The model under review builds one solid part; all positions refer to its coordinate system, in mm. Face numbers are marked on the shaded views. Round coordinates to 2 decimals unless told otherwise and drop trailing zeros.
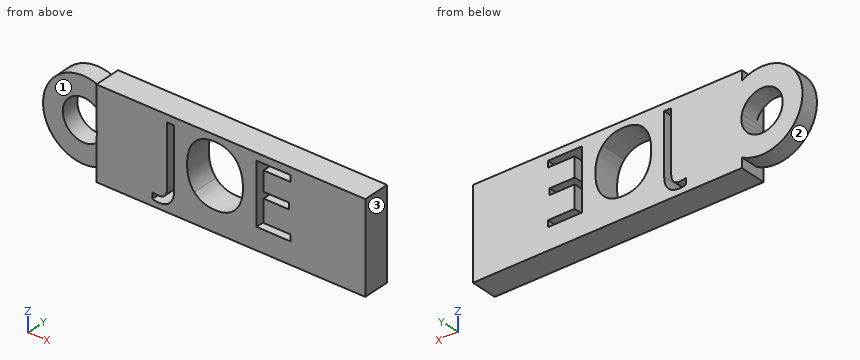
```python
from build123d import *

# Parameters (mm, degrees)
F1_DEPTH = 15
F2_DEPTH = 10


with BuildPart() as f1:
    # F0 (on Front) → F1 (new body)
    with BuildSketch(Plane.XZ):
        with BuildLine():
            Line((-150, 0), (0, 0))
            Line((0, 0), (0, 50))
            Line((0, 50), (-150, 50))
            Line((-150, 50), (-150, 44.6036947758))
            Line((-150, 44.6036947758), (-150, 27.5289733242))
            ThreePointArc((-150, 27.5289733242), (-149.78939418, 26.2722736231), (-149.7189046187, 25))
            ThreePointArc((-149.7189046187, 25), (-149.78939418, 23.7277263769), (-150, 22.4710266758))
            Line((-150, 22.4710266758), (-150, 5.3963052242))
            Line((-150, 5.3963052242), (-150, 0))
        make_face()
        with BuildLine():
            add(Edge.make_bspline(
                [(-108.8792543819, 5.5825479955), (-111.1049800612, 3.1602165479), (-115.2819252527, 3.1602165479)],
                knots=[0, 0, 0, 1, 1, 1], degree=2))
            add(Edge.make_bspline(
                [(-115.2819252527, 3.1602165479), (-117.4557173328, 3.1602165479), (-118.7095427989, 3.7834197381)],
                knots=[0, 0, 0, 1, 1, 1], degree=2))
            Line((-118.7095427989, 3.7834197381), (-118.7095427989, 7.1442655139))
            add(Edge.make_bspline(
                [(-118.7095427989, 7.1442655139), (-117.0625057962, 6.6842822068), (-115.2819252527, 6.6842822068)],
                knots=[0, 0, 0, 1, 1, 1], degree=2))
            add(Edge.make_bspline(
                [(-115.2819252527, 6.6842822068), (-112.9820087174, 6.6842822068), (-111.7875359362, 8.0753607564)],
                knots=[0, 0, 0, 1, 1, 1], degree=2))
            add(Edge.make_bspline(
                [(-111.7875359362, 8.0753607564), (-110.593063155, 9.4664393059), (-110.593063155, 12.0853765219)],
                knots=[0, 0, 0, 1, 1, 1], degree=2))
            Line((-110.593063155, 12.0853765219), (-110.593063155, 45.9831786178))
            Line((-110.593063155, 45.9831786178), (-106.6535287026, 45.9831786178))
            Line((-106.6535287026, 45.9831786178), (-106.6535287026, 12.4118162882))
            add(Edge.make_bspline(
                [(-106.6535287026, 12.4118162882), (-106.6535287026, 8.0048794432), (-108.8792543819, 5.5825479955)],
                knots=[0, 0, 0, 1, 1, 1], degree=2))
        make_face(mode=Mode.SUBTRACT)
        with BuildLine():
            add(Edge.make_bspline(
                [(-72.3402578132, 41.8804242823), (-68.2375034777, 37.2434957837), (-68.2375034777, 29.0825016263)],
                knots=[0, 0, 0, 1, 1, 1], degree=2))
            add(Edge.make_bspline(
                [(-68.2375034777, 29.0825016263), (-68.2375034777, 20.9437647256), (-72.3550959844, 16.2808694274)],
                knots=[0, 0, 0, 1, 1, 1], degree=2))
            add(Edge.make_bspline(
                [(-72.3550959844, 16.2808694274), (-76.4726884911, 11.6179741293), (-83.7953259761, 11.6179741293)],
                knots=[0, 0, 0, 1, 1, 1], degree=2))
            add(Edge.make_bspline(
                [(-83.7953259761, 11.6179741293), (-91.2811833442, 11.6179741293), (-95.3505517945, 16.1992594859)],
                knots=[0, 0, 0, 1, 1, 1], degree=2))
            add(Edge.make_bspline(
                [(-95.3505517945, 16.1992594859), (-99.4199202448, 20.7805448424), (-99.4199202448, 29.1270161398)],
                knots=[0, 0, 0, 1, 1, 1], degree=2))
            add(Edge.make_bspline(
                [(-99.4199202448, 29.1270161398), (-99.4199202448, 37.4067156669), (-95.3394231661, 41.9620342239)],
                knots=[0, 0, 0, 1, 1, 1], degree=2))
            add(Edge.make_bspline(
                [(-95.3394231661, 41.9620342239), (-91.2589260874, 46.5173527809), (-83.7508114625, 46.5173527809)],
                knots=[0, 0, 0, 1, 1, 1], degree=2))
            add(Edge.make_bspline(
                [(-83.7508114625, 46.5173527809), (-76.4430121488, 46.5173527809), (-72.3402578132, 41.8804242823)],
                knots=[0, 0, 0, 1, 1, 1], degree=2))
        make_face(mode=Mode.SUBTRACT)
        Polygon((-41.7884633219, 15.6094421808), (-41.7884633219, 12.0853765219), (-60.6848743392, 12.0853765219), (-60.6848743392, 45.9831786178), (-41.7884633219, 45.9831786178), (-41.7884633219, 42.4813702157), (-56.7453398869, 42.4813702157), (-56.7453398869, 31.5604762159), (-42.6935917648, 31.5604762159), (-42.6935917648, 28.0809250706), (-56.7453398869, 28.0809250706), (-56.7453398869, 15.6094421808), align=None, mode=Mode.SUBTRACT)
    extrude(amount=F1_DEPTH)

    # F0 (on Front) → F2 (join)
    with BuildSketch(Plane.XZ):
        with BuildLine():
            ThreePointArc((-150, 44.6036947758), (-183.8311862448, 25), (-150, 5.3963052242))
            Line((-150, 5.3963052242), (-150, 22.4710266758))
            ThreePointArc((-150, 22.4710266758), (-172.7527967389, 25), (-150, 27.5289733242))
            Line((-150, 27.5289733242), (-150, 44.6036947758))
        make_face()
    extrude(amount=F2_DEPTH)


solid = f1.part
```
(1) Draft analysis for pull direction X (two halves, no side actions). For the marked faces 1, 2 and 3, state which applies: pulls with the +X half, pulls with the -X half, needs draft (parallel to the pull), parting line crosses it, or undercut.
Data:
face 1: needs draft
face 2: undercut
face 3: pulls with the +X half
(2) Insertion check: pin 1 (4 mm diameter, centred on y = -11, z = 43.5, fed in from -X); pin 2 (4.5 mm diameter, centred on y = -8, z = 9.5, fed in from -X); pin 3 (4 mm diameter, centred on y = -6.5, z = 7, fed in from -X). Each pin has a flat end and moves straight along its axis. Give the tip position at first contact, or say it passes through.
Data:
pin 1: stops at x = -176.38
pin 2: stops at x = -179.54
pin 3: stops at x = -177.19
(3) To check wall thickness, follow probe 1 along Z at (x, y) = (-56, -9.5); probe 2 along X at (y, z) = (-3.5, 40); probe 3 along Z at (x, y) = (-84.5, -12.25). State the ranges of each line that lie inside material, in increasing order.
Data:
probe 1: z = 0 to 12.09, 15.61 to 28.08, 31.56 to 42.48, 45.98 to 50
probe 2: x = -178.13 to -110.59, -106.65 to -96.8, -70.93 to -60.68, -56.75 to 0
probe 3: z = 0 to 11.63, 46.51 to 50
(4) Consider section A-A (y = -2). State how many separate pieces and enclosed holes the cut face has, and give its area (3 significant figures).
Data:
separate pieces: 1
enclosed holes: 4
area: 7,000 mm2
